```python
from build123d import *

# Parameters (mm, degrees)
SCHIZZO1_W                   = 76.9
SCHIZZO1_H                   = 60
ESTRUSIONE_ESTRUSIONE1_DEPTH = 3
RIVOLUZIONE2_ANGLE           = 180
SCHIZZO3_W                   = 82.857519441
SCHIZZO3_H                   = 19.07586099
TAGLIO_ESTRUSIONE1_DEPTH     = 87.921415247
SCHIZZO8_W                   = 15.498915434
SCHIZZO8_H                   = 3
SCHIZZO5_W                   = 31.459803045
SCHIZZO5_H                   = 71.75772661
TAGLIO_ESTRUSIONE2_DEPTH     = 86.17399838
SCHIZZO6_W                   = 24.433814687
SCHIZZO6_H                   = 10
TAGLIO_ESTRUSIONE3_DEPTH     = 52.984637154
SCHIZZO7_R                   = 1.75
TAGLIO_ESTRUSIONE4_DEPTH     = 52.984637154


with BuildPart() as part:
    # Schizzo1 → Estrusione-Estrusione1 (new body)
    with BuildSketch(Plane.XY):
        Rectangle(SCHIZZO1_W, SCHIZZO1_H)
    extrude(amount=ESTRUSIONE_ESTRUSIONE1_DEPTH)

    # Schizzo2 → Rivoluzione2 (revolve)
    with BuildSketch(Plane(origin=(0, 0, -7), x_dir=(-1, 0, 0), z_dir=(0, 0, -1))):
        Polygon((-1.948915434, 34.651441941), (-1.948915434, -22), (23.55, -22), (23.55, -9), (15.95, -9), (15.95, 9), (12.05, 9), (12.05, 17.8), (16.55, 17.8), (16.55, 34.651441941), align=None)
    revolve(axis=Axis((4.45, 39.663918646, -7), (0, 1, 0)), revolution_arc=RIVOLUZIONE2_ANGLE)

    # Schizzo3 → Taglio-Estrusione1 (cut, through all)
    with BuildSketch(Plane(origin=(38.45, 0, 0), x_dir=(0, 0, -1), z_dir=(1, 0, 0))):
        with Locations((-0.84285559, 39.537930495)):
            Rectangle(SCHIZZO3_W, SCHIZZO3_H)
    extrude(amount=-TAGLIO_ESTRUSIONE1_DEPTH, mode=Mode.SUBTRACT)

    # Schizzo8 → Taglia-Rivoluzione1 (revolve, cut)
    with BuildSketch(Plane(origin=(0, 0, -7), x_dir=(-1, 0, 0), z_dir=(0, 0, -1))):
        Polygon((13.55, 20.8), (13.55, 27), (-1.948915434, 27), (-1.948915434, -19), (20.55, -19), (20.55, -12), (12.95, -12), (12.95, 6), (9.05, 6), (9.05, 20.8), align=None)
        with Locations((5.800542283, 28.5)):
            Rectangle(SCHIZZO8_W, SCHIZZO8_H)
    revolve(axis=Axis((4.45, 30, -7), (0, -1, 0)), mode=Mode.SUBTRACT)

    # Schizzo5 → Taglio-Estrusione2 (cut, through all)
    with BuildSketch(Plane(origin=(38.45, 0, 0), x_dir=(0, 0, -1), z_dir=(1, 0, 0))):
        with Locations((15.729901523, 13.341257692)):
            Rectangle(SCHIZZO5_W, SCHIZZO5_H)
    extrude(amount=-TAGLIO_ESTRUSIONE2_DEPTH, mode=Mode.SUBTRACT)

    # Schizzo6 → Taglio-Estrusione3 (cut, through all)
    with BuildSketch(Plane.XY.offset(3)):
        with Locations((-26.233092657, 25)):
            Rectangle(SCHIZZO6_W, SCHIZZO6_H)
    extrude(amount=-TAGLIO_ESTRUSIONE3_DEPTH, mode=Mode.SUBTRACT)

    # Schizzo7 → Taglio-Estrusione4 (cut, through all)
    with BuildSketch(Plane.XY.offset(3)):
        with Locations((-33.45, 15)):
            Circle(SCHIZZO7_R)
        with Locations((-33.45, -15)):
            Circle(SCHIZZO7_R)
        with Locations((33.45, -25)):
            Circle(SCHIZZO7_R)
        with Locations((35.2, 25)):
            Circle(SCHIZZO7_R)
    extrude(amount=-TAGLIO_ESTRUSIONE4_DEPTH, mode=Mode.SUBTRACT)


solid = part.part
```
For this review, take the finished solid that the model builds, in its own axes (mm). A direction names the side the tool comes from. Round coordinates to 2 decimals unless told otherwise and drop trailing zeros. Write each loop counter-clockwise with the first axis right and the second up, starting at its lowest first coordinate (ties: lowest second). Pieces come first, ordered by that corner, then holes. Notation, with made-up numbers: (17, 65) - (37, 65) arc R15 cw to (37, 76) - close; hole circle Ø9 at (21, -8.5). An arc over 180 degrees is marked (long way). Put each result on its own line as item: value.
Q1. Wall thickness on probe 1 along Y at (x, z) = (1, 11.5); probe 2 along Y at (x, z) = (-33.45, 0.8); probe 3 along Y at (x, z) = (14.5, 12): over which ranges is each line inside the solid? List them lowest first.
Solved:
probe 1: y = -22 to -19, -12 to 9, 17.8 to 30
probe 2: y = -30 to -16.75, -13.25 to 13.25, 16.75 to 20
probe 3: y = -22 to -19, -12 to -9
Q2. We need section A-A (x = -33.45). Give the boundary of the cut face in (y, z).
Solved:
outline: (-30, 0) - (-16.75, 0) - (-16.75, 3) - (-30, 3) - close; (-13.25, 0) - (13.25, 0) - (13.25, 3) - (-13.25, 3) - close; (16.75, 0) - (20, 0) - (20, 3) - (16.75, 3) - close
Q3. Mouldability with a two-part tool opening along X and no side actions: class faces 1 (the face through (5, 6, 7)), 2 (the face through (-9, 7, 0)), 3 (the face through (-38.45, -5, 1)) as released by +X, released by -X, zero draft, split by the parting line, or undercut.
Solved:
face 1: undercut
face 2: zero draft
face 3: released by -X
Q4. Insertion check: pin 1 Ø1.5 at (x, y) = (12.5, 4.5) entering from +Z; pin 2 Ø1 at (x, y) = (-13.5, -18.5) entering from +Z; pin 3 Ø5 at (x, z) = (-13.5, 10) entering from -Y; pin 4 Ø3 at (x, y) = (-33.45, 15) entering from -Z. Each pin has a flat end and moves straight along its axis. Give the tip position at first contact, or say it passes through.
Solved:
pin 1: stops at z = 12.05
pin 2: stops at z = 14.9
pin 3: stops at y = -22
pin 4: passes through
Q5. We need section D-D (x = 3). Give the boundary of the cut face in (y, z).
Solved:
outline: (-30, 0) - (-19, 0) - (-19, 17.96) - (-12, 17.96) - (-12, 10.34) - (6, 10.34) - (6, 6.42) - (20.8, 6.42) - (20.8, 10.94) - (30, 10.94) - (30, 13.95) - (17.8, 13.95) - (17.8, 9.44) - (9, 9.44) - (9, 13.35) - (-9, 13.35) - (-9, 20.96) - (-22, 20.96) - (-22, 3) - (-30, 3) - close
Q6. We need section B-B (y = -25). Give the boundary of the cut face in (x, z), and give its area (3 significant figures).
Solved:
outline: (-38.45, 0) - (31.7, 0) - (31.7, 3) - (-38.45, 3) - close; (35.2, 0) - (38.45, 0) - (38.45, 3) - (35.2, 3) - close
area: 220 mm2
Q7. Machinability: for faces 4 (the face through (5, 9, 11)), 5 (the face through (4, -22, 10)), 6 (the face through (33.91, 26.18, 1.52)), 7 (the face through (4.7, -2.9, 10.4)), which of the approach directions +Z, -Z, +X, -X, +Y, -Y give a long, thin tool a straight path to every point of the face, cutting with its end or side? Answer none if there is none.
Solved:
face 4: +Z
face 5: +Z, +X, -X, -Y
face 6: +Z, -Z
face 7: -Z
Q8. We need section C-C (y = -2.5). Give the boundary of the cut face in (x, z), and give its area (3 significant figures).
Solved:
outline: (-38.45, 0) - (-11.48, 0) arc R17.4 cw to (20.38, 0) - (38.45, 0) - (38.45, 3) - (22.23, 3) arc R20.4 ccw to (-13.33, 3) - (-38.45, 3) - close
area: 255 mm2
